Autodesk Inventor part; units mm, degrees
ref_plane "Work Plane1" through (4.3209, 15, 0) normal (0, 1, 0) x (1, 0, 0)
ref_plane "YZ Plane" through (0, 0, 0) normal (1, 0, 0) x (0, 1, 0)
ref_plane "XZ Plane" through (0, 0, 0) normal (0, 1, 0) x (-1, 0, 0)
sketch "Sketch2" plane through (0, 0, 0) normal (0, 1, 0) x (-1, 0, 0)
  line L0 (0, 0) -> (23.273, 0)
  line L1 (23.273, 0) -> (23.273, -37.9053)
  line L2 (23.273, -37.9053) -> (0, -37.9053)
  line L3 (0, -37.9053) -> (0, 0)
  line L4 (26.75, 0) -> (-5, 0)
  line L5 (-5, 0) -> (-5, -37.9053)
  line L6 (-5, -37.9053) -> (26.75, -37.9053)
  line L7 (26.75, -37.9053) -> (26.75, 0)
  point P0 (0, -37.9053)
  dimension "d21" = 37.9053
  dimension "d22" = 23.273
  dimension "d36" = 5
  dimension "d37" = 31.75
extrude "Extrusion1" add sketch "Sketch2" along normal blind 15
sketch "Sketch6" plane through (-26.75, 0, 0) normal (0, 0, 1) x (1, 0, 0)
  line L0 (31.75, 0) -> (31.75, 15)
  line L1 (31.75, 0) -> (31.75, 15)
  line L2 (31.75, 0) -> (0, 0)
  line L3 (30.3918, 0) -> (30.3918, 15)
  line L4 (31.75, 15) -> (0, 15)
  line L5 (30.3918, 15) -> (55.3918, 15) construction
  line L6 (0, 0) -> (0, 15)
  line L7 (0, 0) -> (0, 0.5)
  line L8 (30.3918, 15) -> (9.894, 0)
  point P0 (26.75, 0)
  dimension "d38" = 1.3582
  dimension "d41" = 0.5
  dimension "d96" = 25.4
  dimension "d97" = 53.804
extrude "Extrusion2" cut sketch "Sketch6" against normal up to surface (37.9053 mm away) contours L8 L2 L6 L4
sketch "Sketch8" plane through (0, 0, 0) normal (0, -1, 0) x (1, 0, 0)
  line L0 (-26.75, -37.9053) -> (-26.75, 0)
  line L1 (-26.75, -10.922) -> (3, -10.922)
  line L2 (3, -10.922) -> (3, -26.9833)
  line L3 (3, -26.9833) -> (-26.75, -26.9833)
  line L4 (-26.75, -26.9833) -> (-26.75, -10.922)
  line L5 (-26.75, 0) -> (5, 0)
  line L6 (5, -37.9053) -> (-26.75, -37.9053)
  line L7 (5, 0) -> (5, -37.9053)
  point P0 (0, 0)
  point P1 (-26.75, -26.9833)
  dimension "d44" = 10.922
  dimension "d45" = 10.922
  dimension "d46" = 2
extrude "Extrusion3" cut sketch "Sketch8" against normal blind 25.4 contours L0 L1 L2 L3
ref_plane "Work Plane1" through (4.3209, 15, 0) normal (0, 1, 0) x (1, 0, 0)
sketch "Sketch12" plane through (0, 0, 0) normal (0, -1, 0) x (1, 0, 0)
  line L0 (3.6418, 0) -> (-26.75, 0)
  line L1 (-26.75, 0) -> (0, 0)
  line L2 (0, 0) -> (0, -5)
  line L3 (0, -5) -> (-26.75, -5)
  line L4 (-26.75, -5) -> (-26.75, 0)
  line L5 (-26.75, -37.9053) -> (0, -37.9053)
  line L6 (0, -37.9053) -> (0, -32.9053)
  line L7 (0, -32.9053) -> (-26.75, -32.9053)
  line L8 (-26.75, -32.9053) -> (-26.75, -37.9053)
  line L9 (5, 0) -> (0, 0)
  line L10 (0, 0) -> (0, -1)
  line L11 (0, -1) -> (5, -1)
  line L12 (5, -1) -> (5, 0)
  line L13 (5, 0) -> (5, -37.9053)
  line L14 (5, -37.9053) -> (0, -37.9053)
  line L15 (0, -37.9053) -> (0, -36.9053)
  line L16 (0, -36.9053) -> (5, -36.9053)
  line L17 (5, -36.9053) -> (5, -37.9053)
  line L18 (5, -37.9053) -> (-26.75, -37.9053)
  point P0 (0, -37.9053)
  dimension "d69" = 5
  dimension "d70" = 5
  dimension "d73" = 1
  dimension "d74" = 1
  dimension "d75" = 0
extrude "Extrusion6" cut sketch "Sketch12" along normal through all both and the other way through all
sketch "Sketch13" plane through (0, 0, -36.9053) normal (-1, 0, 0) x (0, 0, 1)
  circle A0 centre (2, 3.9204) radius 1.5
  circle A1 centre (33.9053, 3.9204) radius 1.5
  line L0 (35.9053, 0) -> (31.9053, 0)
  line L1 (31.9053, 7.8408) -> (35.9053, 7.8408)
  line L2 (35.9053, 12.335) -> (35.9053, 0)
  line L3 (31.9053, 2) -> (31.9053, 7.8408)
  line L4 (0, 0) -> (0, 12.335)
  line L5 (0, 7.8408) -> (4, 7.8408)
  line L6 (4, 0) -> (0, 0)
  point P0 (36.9053, 0)
  point P1 (35.9053, 8.636)
  point P2 (0, 8.636)
  dimension "d80" = 3
  dimension "d81" = 3
  dimension "d82" = 7.8408
  dimension "d83" = 3.9204
  dimension "d84" = 4
  dimension "d85" = 2
  dimension "d86" = 2
  dimension "d87" = 3.9204
  dimension "d88" = 31.9053
  dimension "d148" = 3.9204
extrude "Extrusion7" cut sketch "Sketch13" against normal blind 25.4
sketch "Sketch15" plane through (3, 14.5303, -10.922) normal (-0.5905512, 0.8070002, 0) x (0.8070002, 0.5905512, 0)
  circle A0 centre (-20.3372, -2.4315) radius 1.1146
  circle A1 centre (-7.798, 18.5871) radius 1.229
  line L0 (-20.3372, -2.4315) -> (-20.3372, 18.5871)
  line L1 (-20.3372, 18.5871) -> (-7.798, 18.5871)
  line L2 (-7.798, 18.5871) -> (-7.798, -2.4315)
  line L3 (-7.798, -2.4315) -> (-20.3372, -2.4315)
  line L4 (-12.87, 2.62) -> (-12.87, 13.4413)
  line L5 (-12.87, 13.4413) -> (-2.4234, 13.4413)
  line L6 (-2.4234, 13.4413) -> (-2.4234, 2.62)
  line L7 (-2.4234, 2.62) -> (-12.87, 2.62)
  line L8 (-22.1086, -4.4694) -> (-22.1086, 20.5306)
  line L9 (-22.1086, 20.5306) -> (1.8914, 20.5306)
  line L10 (1.8914, 20.5306) -> (1.8914, -4.4694)
  line L11 (1.8914, -4.4694) -> (-22.1086, -4.4694)
  line L12 (-3.7175, 21.9833) -> (-24.6047, 21.9833)
  line L13 (-24.6047, -5.922) -> (-3.7175, -5.922)
  circle A2 centre (-20.3372, 18.5871) radius 1.1245
  line L14 (0, 16.0613) -> (0, 0)
  line L15 (1.8914, -9.922) -> (1.8914, 25.9833)
  circle A3 centre (-7.798, -2.4315) radius 1.1245
  point P0 (-11.0019, -10.922)
  dimension "d107" = 21.0186
  dimension "d108" = 12.5392
  dimension "d110" = 25
  dimension "d111" = 24
  dimension "d112" = 4.3148
  dimension "d113" = 9.2386
  dimension "d114" = 7.0893
  dimension "d115" = 7.0893
  dimension "d117" = 1.9436
  dimension "d118" = 2.0378
  dimension "d119" = 1.7714
  dimension "d120" = 9.6893
  dimension "d122" = 1.4526
  dimension "d123" = 1.4526
  dimension "d124" = 2.249
  dimension "d133" = 0
  dimension "d134" = 2.249
hole "Hole3" at (-13.4121, 2.5202, -8.4905) at (-3.293, 9.9252, -8.4905) at (-3.293, 9.9252, -29.5091) at (-13.4121, 2.5202, -29.5091) direction (0.5905512, -0.8070002, 0) diameter 2.1211 depth 7.1 tip angle 118 countersink diameter 2.125 countersink angle 90
chamfer "Chamfer3" distance 2 distance2 2 1 edges at (3, 0, -18.9526) measured on face at (-2.4276, 0, -8.2115)
equation "\"d83\" = 0.5 * d82"
equation "\"d85\" = 0.5 * d84"
equation "\"d86\" = d85"
equation "\"d87\" = d83"
equation "\"d115\" = d114"
equation "\"d122\" = d123"
properties part number "Camera Angle"
Build history of the part. All positions in model axes, mm. A direction names the side the tool comes from. Coordinates: 2 decimals unless noted, no trailing zeros. Order: outer loops, then holes, each group sorted by start corner. A loop starts at its lowest first (then second) coordinate and runs counter-clockwise, first axis right, second up. Notation, with made-up numbers: M 22.25,-27.75 L 34.25,-27.75 A32 ccw 34.25,8.25 Z; hole C 64,75 d10. An arc over 180 degrees is marked long. One line per question, with ' | ' between items. Start each with the question number.
1. Cut at A-A (x = 2.5). Write the cut outline in (y, z).
2. Flat gauge pins, fed straight in: P1, Ø6, axis at x = -7, y = 4, coming from the +Z side; P2, Ø2, axis at y = 6, z = -34, coming from the -X side; P3, Ø2.5, axis at y = 3.92, z = -34.91, coming from the +X side; P4, Ø3.5, axis at x = -6, y = 6.5, coming from the -Z side. Where does each tip first touch, or does it go through?
3. Cut at D-D (y = 11.5). Write the cut outline in (x, z).
4. Cut at C-C (x = -4.75). Write the cut outline in (y, z).
5. Cut at B-B (z = -3). Write the cut outline in (x, y), plus the area to 3 significant figures.
6. Tool access for faces 4 (the face through (4, 1, -19)), 5 (the face through (1.154, 3.729, -29.339)), 6 (the face through (-6, 5, -5)), 7 (the face through (-6, 5, -32.905)): list every direction of +Z, -Z, +X, -X, +Y, -Y with a clear straight run to the whole face (end or side of a thin tool).
7. Wall check: line 1 along Z through (x, y) = (-13, 1.75); line 2 along Z through (x, y) = (0.5, 5); line 3 along Z through (x, y) = (2.25, 3.5). Give the ranges that are in metal, low to high. Write a range as [from, to].
8. Mould opens along Y. For faces 1 (the face through (-11.74, 1.83, -29.02)), 2 (the face through (4, 15, -19)), 3 (the face through (-4, 4, -10.922)) say: +Y half, -Y half, draft (parallel to the pull), parting line (faces both ways), or undercut.
The answers:
1) outline: M 0,-36.91 L 14.16,-36.91 L 14.16,-26.98 L 0,-26.98 Z; M 0,-10.92 L 14.16,-10.92 L 14.16,-1 L 0,-1 Z; hole C 3.92,-34.91 d3; hole C 3.92,-3 d3
2) P1: stops at z = -5 | P2: stops at x = 0 | P3: passes through | P4: stops at z = -32.91
3) outline: M -1.14,-32.91 L 0,-32.91 L 0,-36.91 L 5,-36.91 L 5,-1 L 0,-1 L 0,-5 L -1.14,-5 L -1.14,-10.92 L 3,-10.92 L 3,-26.98 L -1.14,-26.98 Z
4) outline: M 0,-32.91 L 8.86,-32.91 L 8.86,-26.98 L 0,-26.98 Z; M 0,-10.92 L 8.86,-10.92 L 8.86,-5 L 0,-5 Z
5) outline: M 0,0 L 5,0 L 5,2.42 L 0,2.42 Z; M 0,5.42 L 5,5.42 L 5,15 L 3.64,15 L 0,12.33 Z | area: 55.1 mm2
6) face 4: -X, -Y | face 5: none | face 6: +Z, -X, +Y, -Y | face 7: -Z, -X, +Y, -Y
7) line 1: z = [-32.91, -30.56], [-28.46, -26.98], [-10.92, -9.54], [-7.44, -5] | line 2: z = [-36.91, -35.95], [-33.86, -30.56], [-28.46, -26.98], [-10.92, -9.54], [-7.44, -4.04], [-1.96, -1] | line 3: z = [-36.91, -36.35], [-33.47, -26.98], [-10.92, -4.44], [-1.56, -1]
8) face 1: undercut | face 2: +Y half | face 3: draft
